Read the model definition and answer for the solid it produces. Units are mm, in the model's axes. A direction names the side the tool comes from. Coordinates: 2 decimals unless noted, no trailing zeros. Loops run counter-clockwise (first coordinate to the right, second up) from the corner with the lowest first, then second, coordinate; pieces in that order, holes last. Notation, with made-up numbers: (-6, 8.5) - (29, 8.5) arc R11 cw to (29, 18.5) - close; hole circle Ø2 at (-13.75, -19). An arc over 180 degrees is marked (long way). Use one line per item in the form item = value. Start each with the question number.
1) Consider line 1 (Y direction, x = 0, z = -2.5); line 2 (X direction, y = 0, z = -1.3); line 3 (Y direction, x = 0.5, z = 0.5). Determine where each line is inside the solid, lowest interval first.
2) Which of the six approach directions +Z, -Z, +X, -X, +Y, -Y give full straight-line access (tool end or side, diameter ignored) to faces 1 (the face through (0, 18, 1.27)), 2 (the face through (0, 18, -1.27)), 3 (the face through (-3.78, 2.9, -2.72))?
3) Each of these flat-tipped pins is pushed along its axis until it touches: P1, Ø4, axis at x = 1.5, y = 28, coming from the -Z side; P2, Ø5.5, axis at x = 0, y = 0, coming from the -Z side; P3, Ø2, axis at x = 2.5, z = 1, coming from the -Y side. Where does it stop, or does it pass through?
4) A cutting plane is placed at B-B (y = 25.4). Give the vertices of the cut face in (x, z) (3 decimals), and give its area (3 significant figures).
5) A cutting plane is placed at C-C (z = -3.75). Give the vertices of the cut face in (x, y), and give its area (3 significant figures).
6) The mould has two halves that part along X. Classify faces 4 (the face through (3, 4, -2.273)), 5 (the face through (0.1, 32.5, 0)), 6 (the face through (-0.633, 2.852, -1.953)), 7 (the face through (0, 0, 0.622)): released by +X, released by -X, zero draft, split by the parting line, or undercut.
from build123d import *

# Parameters (mm, degrees)
F1_DEPTH  = 1.27
F2_W      = 12.7
F2_H      = 1.0033
F3_DEPTH  = 6.5
F5_DEPTH  = 4.5476
F6_R      = 4.7625
F7_DEPTH  = 2.1844
F8_SIZE   = 1.27
F9_R      = 2.921
F10_DEPTH = 5.08
F11_R     = 0.635
F12_DEPTH = 25.4


# Not quite as in the source:
# - after a boolean that leaves OpenCascade's solid faulty, fix() repairs it


with BuildPart() as f1:
    # F0 (on Top) → F1 (new body, symmetric)
    with BuildSketch(Plane.XY):
        with BuildLine():
            ThreePointArc((-6.465126425, 0.6724137931), (-0.3366587573, -6.4912757514), (6.5, 0))
            ThreePointArc((6.5, 0), (6.4912757514, 0.3366587573), (6.465126425, 0.6724137931))
            ThreePointArc((6.465126425, 0.6724137931), (0, 6.5), (-6.465126425, 0.6724137931))
        make_face()
        with BuildLine():
            ThreePointArc((-6.465126425, 0.6724137931), (0, 6.5), (6.465126425, 0.6724137931))
            Line((6.465126425, 0.6724137931), (3.4812219211, 29.3620689655))
            ThreePointArc((3.4812219211, 29.3620689655), (3.4953023277, 29.1812777924), (3.5, 29))
            ThreePointArc((3.5, 29), (-0.1812777924, 25.5046976723), (-3.4812219211, 29.3620689655))
            Line((-3.4812219211, 29.3620689655), (-6.465126425, 0.6724137931))
        make_face()
        with BuildLine():
            ThreePointArc((3.5, 29), (3.4953023277, 29.1812777924), (3.4812219211, 29.3620689655))
            ThreePointArc((3.4812219211, 29.3620689655), (0, 32.5), (-3.4812219211, 29.3620689655))
            ThreePointArc((-3.4812219211, 29.3620689655), (-0.1812777924, 25.5046976723), (3.5, 29))
        make_face()
    extrude(amount=F1_DEPTH, both=True)

    # F2 (on Right) → F3 (join, symmetric)
    with BuildSketch(Plane.YZ):
        with Locations((-0.15, -1.77165)):
            Rectangle(F2_W, F2_H)
        with Locations((-0.15, 1.77165)):
            Rectangle(F2_W, F2_H)
        Polygon((8.74, 1.27), (6.2, 2.2733), (6.2, 1.27), align=None)
        Polygon((8.74, -1.27), (6.2, -1.27), (6.2, -2.2733), align=None)
    extrude(amount=F3_DEPTH, both=True)

    # F4 (on face) → F5 (cut, through all)
    with BuildSketch(Plane.XY.offset(2.2733)):
        Polygon((5.6260467402, 8.74), (5.8902227087, 6.2), (6.5, 6.2), (6.5, 8.74), align=None)
        with BuildLine():
            Line((6.5, 6.2), (5.8902227087, 6.2))
            Line((5.8902227087, 6.2), (6.465126425, 0.6724137931))
            ThreePointArc((6.465126425, 0.6724137931), (6.4912757514, 0.3366587573), (6.5, 0))
            Line((6.5, 0), (6.5, 6.2))
        make_face()
        with BuildLine():
            ThreePointArc((6.5, 0), (4.5961940777, -4.5961940777), (0, -6.5))
            Line((0, -6.5), (6.5, -6.5))
            Line((6.5, -6.5), (6.5, 0))
        make_face()
        with BuildLine():
            ThreePointArc((0, -6.5), (-4.5961940777, -4.5961940777), (-6.5, 0))
            Line((-6.5, 0), (-6.5, -6.5))
            Line((-6.5, -6.5), (0, -6.5))
        make_face()
        Polygon((-6.5, 6.2), (-5.8902227087, 6.2), (-5.6260467402, 8.74), (-6.5, 8.74), align=None)
        with BuildLine():
            ThreePointArc((-6.5, 0), (-6.4912757514, 0.3366587573), (-6.465126425, 0.6724137931))
            Line((-6.465126425, 0.6724137931), (-5.8902227087, 6.2))
            Line((-5.8902227087, 6.2), (-6.5, 6.2))
            Line((-6.5, 6.2), (-6.5, 0))
        make_face()
    extrude(amount=-F5_DEPTH, mode=Mode.SUBTRACT)

    add(f1.part.fix(), mode=Mode.REPLACE)

    # F6 (on face) → F7 (join)
    with BuildSketch(Plane(origin=(0, 0, -2.2733), x_dir=(1, 0, 0), z_dir=(0, 0, -1))):
        Circle(F6_R)
    extrude(amount=F7_DEPTH)

    # F8
    f8_edges = [f1.edges().sort_by_distance(p)[0] for p in [
        (-4.7625, 0, -4.4577),
    ]]
    chamfer(f8_edges, length=F8_SIZE)

    # F9 (on face) → F10 (cut)
    with BuildSketch(Plane(origin=(0, 0, -4.4577), x_dir=(1, 0, 0), z_dir=(0, 0, -1))):
        Circle(F9_R)
    extrude(amount=-F10_DEPTH, mode=Mode.SUBTRACT)

    add(f1.part.fix(), mode=Mode.REPLACE)

    # F11 (on face) → F12 (cut)
    with BuildSketch(Plane.XY.offset(1.27)):
        with Locations((0, 25.4)):
            Circle(F11_R)
    extrude(amount=-F12_DEPTH, mode=Mode.SUBTRACT)


solid = f1.part
Found:
q1.line_1 = -4.76 to -2.92, 2.92 to 4.76
q1.line_2 = -6.5 to -2.92, 2.92 to 6.5
q1.line_3 = -6.48 to -2.88, 2.88 to 25.01, 25.79 to 32.46
q2.face_1 = +Z, +X, -X, +Y
q2.face_2 = -Z, +X, -X, +Y
q2.face_3 = -Z
q3.P1 = -1.27
q3.P2 = 0.62
q3.P3 = -6.32
q4.outline = (-3.893, -1.27) - (-0.635, -1.27) - (-0.635, 1.27) - (-3.893, 1.27) - close; (0.635, -1.27) - (3.893, -1.27) - (3.893, 1.27) - (0.635, 1.27) - close
q4.area = 16.6 mm^2
q5.outline = circle Ø8.4 at (0, 0); hole circle Ø5.84 at (0, 0)
q5.area = 28.6 mm^2
q6.face_4 = zero draft
q6.face_5 = split by the parting line
q6.face_6 = undercut
q6.face_7 = undercut
